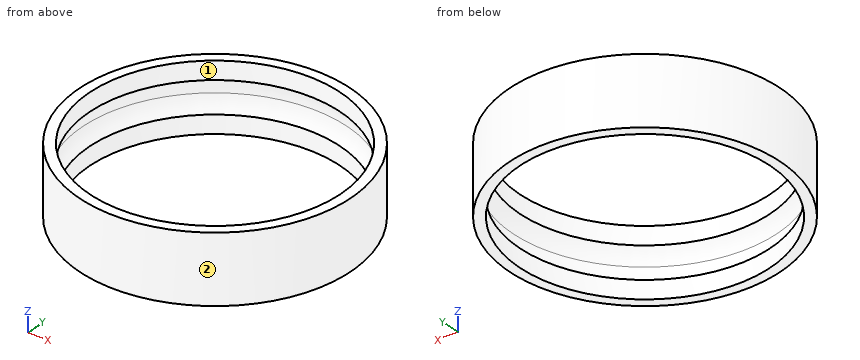
Solid Edge part; units mm, degrees
sketch "Sketch1" plane through (0, 0, 0) normal (1, 0, 0) x (0, 1, 0)
  line L0 (37, 10) -> (37, -10)
  line L1 (37, -10) -> (40, -10)
  line L2 (40, -10) -> (40, 10)
  line L3 (37, 10) -> (40, 10)
  dimension "D1" = 37
  dimension "D2" = 40
revolve "RevolvedProtrusion1" add sketch "Sketch1" angle 360 about axis through (0, 0, -57) along (0, 0, 1)
sketch "Sketch2" plane through (0, 0, 0) normal (0, -1, 0) x (1, 0, 0)
  circle A0 centre (32.5, 0) radius 6.5
revolve "RevolvedCutout1" cut sketch "Sketch2" angle 360 about axis through (0, 0, 54) along (0, 0, -1)
properties material "Polyethylene, low density"
The listing builds one solid part. Answer for the finished solid, in the listing's coordinates (mm). Face numbers are marked on the shaded views. Give positions to 0.01 mm unless a question says otherwise; leave off trailing zeros. Write each loop counter-clockwise with the first axis right and the second up, starting at its lowest first coordinate (ties: lowest second). Pieces come first, ordered by that corner, then holes. Notation, with made-up numbers: (61.5, 81.5) -> (84.5, 81.5) arc R18 ccw to (84.5, 93.5) -> close; hole circle Ø5 at (54, 22). An arc over 180 degrees is marked (long way). Write item = value, one per line. Start each with the question number.
1) Each of these flat-tipped pins is pushed along its axis until it touches: pin 1 (6 mm diameter, centred on y = 21.5, z = 6.5, fed in from +X); pin 2 (12 mm diameter, centred on y = -2.5, z = -0.5, fed in from -X); pin 3 (8 mm diameter, centred on y = 0.5, z = -2, fed in from +X). Where does it stop, or does it pass through?
2) Straight lines are drawn through the part: line 1 along Y through (x, z) = (0, 7.1); line 2 along X through (y, z) = (-25, 7). For each, find the intervals that lie inside material, in ascending order.
3) The part is cut by section D-D, the plane z = -2. Determine the outline of the cut face in (x, y), and give its area (3 significant figures).
4) The part is cut by section C-C, the plane z = -6.75. Determine the outline of the cut face in (x, y).
5) Determine the mould class of the marked faces 1 and 2 for opening direction Y: +Y half, -Y half, draft (parallel to the pull), parting line (faces both ways), or undercut.
6) The part is cut by section A-A, the plane y = 0. Determine the outline of the cut face in (x, z), and give its area (3 significant figures).
Solutions:
q1.pin_1 = 35.46
q1.pin_2 = -40
q1.pin_3 = 40
q2.line_1 = -40 to -37, 37 to 40
q2.line_2 = -31.22 to -27.28, 27.28 to 31.22
q3.outline = circle Ø80 at (0, 0); hole circle Ø77.37 at (0, 0)
q3.area = 325 mm²
q4.outline = circle Ø80 at (0, 0); hole circle Ø74 at (0, 0)
q5.face_1 = undercut
q5.face_2 = parting line
q6.outline = (-40, -10) -> (-37, -10) -> (-37, -4.69) arc R6.5 cw to (-37, 4.69) -> (-37, 10) -> (-40, 10) -> close; (37, -10) -> (40, -10) -> (40, 10) -> (37, 10) -> (37, 4.69) arc R6.5 cw to (37, -4.69) -> close
q6.area = 94.1 mm²
